```python
from build123d import *

# Parameters (mm, degrees)
SALIENTE_EXTRUIR2_DEPTH = 350
CORTAR_EXTRUIR1_DEPTH   = 350
CROQUIS4_W              = 1000
CROQUIS4_H              = 40
CORTAR_EXTRUIR2_DEPTH   = 30


with BuildPart() as part:
    # Croquis2 → Saliente-Extruir2 (new body)
    with BuildSketch(Plane.XY):
        Polygon((0, 0), (741.33697933, 297.624853905), (719.728110413, 351.449167966), (0, 58), (-1288.66302067, 58), (-1288.66302067, 0), align=None)
    extrude(amount=SALIENTE_EXTRUIR2_DEPTH)

    # Croquis3 → Cortar-Extruir1 (cut)
    with BuildSketch(Plane.XY.offset(350)):
        Polygon((-1288.66302067, 30), (-1288.66302067, 0), (-1248.66302067, 0), align=None)
    extrude(amount=-CORTAR_EXTRUIR1_DEPTH, mode=Mode.SUBTRACT)

    # Croquis4 → Cortar-Extruir2 (cut)
    with BuildSketch(Plane(origin=(0, 58, 0), x_dir=(1, 0, 0), z_dir=(0, 1, 0))):
        with Locations((-638.66302067, -87.5)):
            Rectangle(CROQUIS4_W, CROQUIS4_H)
        with Locations((-638.66302067, -262.5)):
            Rectangle(CROQUIS4_W, CROQUIS4_H)
    extrude(amount=-CORTAR_EXTRUIR2_DEPTH, mode=Mode.SUBTRACT)


solid = part.part
```
Check sheet for the modelled part. Datum: model origin and axes. Units: mm. A direction names the side the tool comes from. Round coordinates to 2 decimals unless told otherwise and drop trailing zeros. Loops run counter-clockwise (first coordinate to the right, second up) from the corner with the lowest first, then second, coordinate; pieces in that order, holes last. Notation, with made-up numbers: (53, 46.25) - (58, 46.25) arc R6 ccw to (58, 51.25) - close; hole circle Ø11 at (-0.5, 50). An arc over 180 degrees is marked (long way). Write item = value, one per line. Start each with the question number.
Q1. Section check C-C (z = 263). Record the boundary of the cut face in (x, y), plus the area to 3 significant figures.
Q2. Depth check by flat-ended pin: P1, Ø15, axis at x = -487.5, y = 44, coming from the -Z side; P2, Ø1, axis at y = 60, z = 90, coming from the +X side; P3, Ø4, axis at y = 39.5, z = 51, coming from the +X side; P4, Ø3, axis at y = 106, z = 153.5, coming from the -X side. Enter the tip coordinate at first touch or a pass-through.
Q3. Release check for a two-part mould opening along X. For faces 4 (the face through (-633, 0, 173)), 5 (the face through (-1268.38, 14.79, 177.45)), 6 (the face through (-646, 28, 262)) record: pulls with the +X half, pulls with the -X half, needs draft (parallel to the pull), parting line crosses it, or undercut.
Q4. Section check B-B (z = 168.5). Record the boundary of the cut face in (x, y).
Q5. Access from +Z, -Z, +X, -X, +Y, -Y to the whole of each face (thin tool, end or side, straight path). Record for faces 1 (the face through (-646, 28, 87)), 2 (the face through (-278, 46, 350)), 3 (the face through (-635, 58, 173)).
Q6. Section check A-A (x = -530). Record the boundary of the cut face in (y, z), plus the area to 3 significant figures.
Q7. Thickness scan on L1, parallel to Y at x = -687, z = 223; L2, parallel to Y at x = -212, z = 267.5; L3, parallel to X at y = 89.5, z = 243. Record the ranges inside material, lowest first.
Q8. Section check D-D (y = 228). Record the boundary of the cut face in (x, z), plus the area to 3 significant figures.
Derived:
q1.outline = (-1288.66, 30) - (-1248.66, 0) - (0, 0) - (741.34, 297.62) - (719.73, 351.45) - (0, 58) - (-138.66, 58) - (-138.66, 28) - (-1138.66, 28) - (-1138.66, 58) - (-1288.66, 58) - close
q1.area = 88,200 mm^2
q2.P1 = 0
q2.P2 = 150.7
q2.P3 = 103.37
q2.P4 = 114.05
q3.face_4 = needs draft
q3.face_5 = pulls with the -X half
q3.face_6 = undercut
q4.outline = (-1288.66, 30) - (-1248.66, 0) - (0, 0) - (741.34, 297.62) - (719.73, 351.45) - (0, 58) - (-1288.66, 58) - close
q5.face_1 = +Y
q5.face_2 = +Z, +X, -X, +Y, -Y
q5.face_3 = +Z, -Z, -X, +Y
q6.outline = (0, 0) - (58, 0) - (58, 67.5) - (28, 67.5) - (28, 107.5) - (58, 107.5) - (58, 242.5) - (28, 242.5) - (28, 282.5) - (58, 282.5) - (58, 350) - (0, 350) - close
q6.area = 17,900 mm^2
q7.L1 = 0 to 58
q7.L2 = 0 to 28
q7.L3 = 77.26 to 222.93
q8.outline = (416.95, 0) - (567.91, 0) - (567.91, 350) - (416.95, 350) - close
q8.area = 52,800 mm^2
